Geometry: see drawing. Coordinates: mm, zero at the bounding-box minimum. Coordinates: 2 decimals unless noted, no trailing zeros. Write each loop counter-clockwise with the first axis right and the second up, starting at its lowest first coordinate (ties: lowest second). Pieces come first, ordered by that corner, then holes. Notation, with made-up numbers: (41, 84.5) -> (53, 84.5) arc R31 cw to (53, 119.5) -> close; hole circle Ø6 at (19, 88). An arc over 180 degrees is marked (long way). Use one line per item in the form item = value. Start each with the question number.
(1) Pull-direction query (Z, two-part tool) for the marked faces 1, 2 and 3; classes: released by +Z, released by -Z, zero draft, split by the parting line, or undercut.
(2) Ray query, line 1 along Z through (x, y) = (2.25, 17.25); line 2 along Y through (x, z) = (14.5, 18.75) (1 decimal); line 3 along X through (y, z) = (10.5, 5.25). Return the intervals inside material, ascending.
(3) First-contact query: pin 1 (4 mm diameter, centred on y = 4, z = 10, fed in from -X); pin 2 (4 mm diameter, centred on x = 14.5, z = 11, fed in from +Y) (1 decimal); pin 3 (1.5 mm diameter, centred on y = 13.5, z = 5, fed in from +X). Flat tips, straight axial feed; report the tip coordinate or a pass-through.
(4) Cut plane A-A on z = 13.75. Return the cut outline in (x, y).
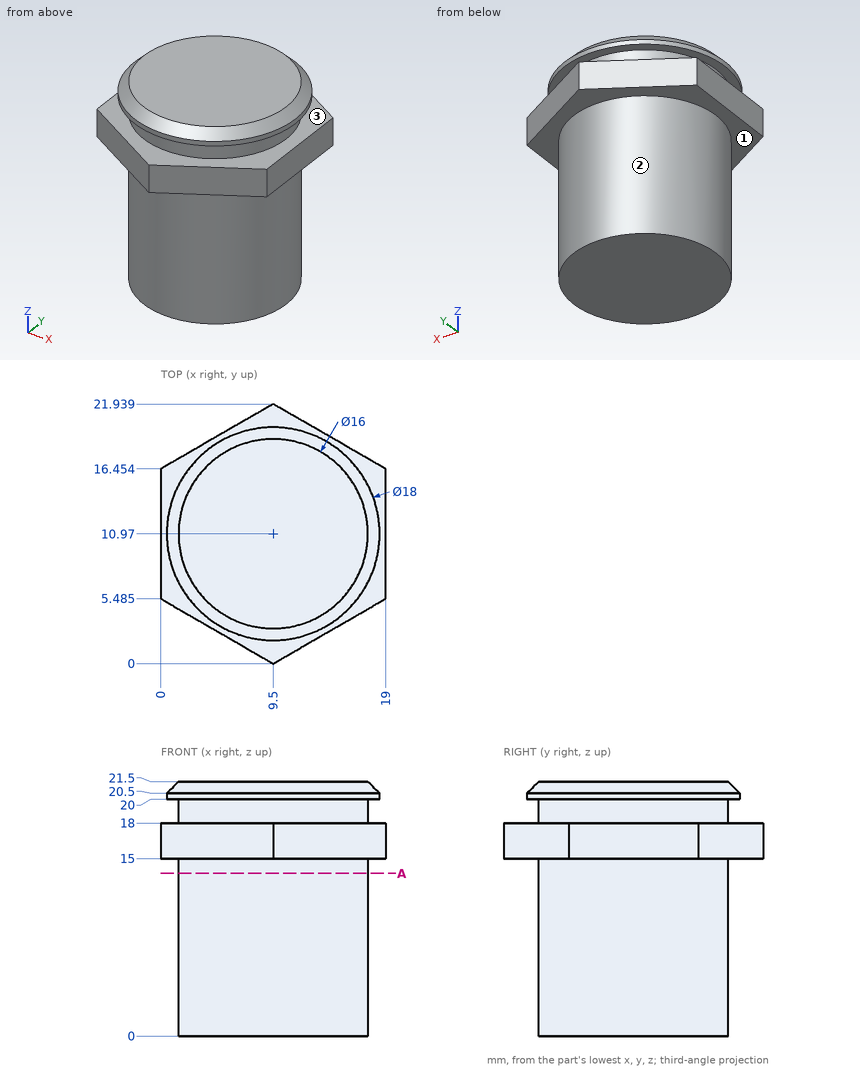
Values:
q1.face_1 = released by -Z
q1.face_2 = zero draft
q1.face_3 = undercut
q2.line_1 = 15 to 18
q2.line_2 = 4.7 to 17.2
q2.line_3 = 1.51 to 17.49
q3.pin_1 = 3.23
q3.pin_2 = 18.4
q3.pin_3 = 17.3
q4.outline = circle Ø16 at (9.5, 10.97)
